Verification items for this drawing (mm, ordinates from the low corner). A direction names the side the tool comes from. Round coordinates to 2 decimals unless told otherwise and drop trailing zeros. Order: outer loops, then holes, each group sorted by start corner. A loop starts at its lowest first (then second) coordinate and runs counter-clockwise, first axis right, second up. Notation, with made-up numbers: (63, 68) -> (78, 68) arc R16 cw to (78, 73) -> close; hole circle Ø2 at (-5, 74.25). An arc over 180 degrees is marked (long way). Answer in a Markdown table with one row per item. Add a question column.
1. Material ranges on L1, parallel to X at y = 76, z = 26.5; L2, parallel to Y at x = 58, z = 7, recorded low to high. Write a range as from..to.
2. Sectioned sample at C-C, the plane z = 15. Record the boundary of the cut face in (x, y), then the cut area to 3 significant figures.
3. Depth check by flat-ended pin: P1, Ø2, axis at y = 63, z = 41, coming from the -X side; P2, Ø6.5, axis at y = 59.14, z = 20.86, coming from the +X side; P3, Ø8, axis at x = 93.5, y = 37, coming from the -Z side. Enter the tip coordinate at first touch or a pass-through.
4. Sectioned sample at D-D, the plane x = 78. Record the boundary of the cut face in (y, z).
5. Access from +Z, -Z, +X, -X, +Y, -Y to the whole of each face (thin tool, end or side, straight path). Record for the marked faces 1 and 2.
6. Sectioned sample at A-A, the plane z = 35. Record the boundary of the cut face in (x, y), then the cut area to 3 significant figures.
7. Sectioned sample at B-B, the plane y = 51.5. Record the boundary of the cut face in (x, z).
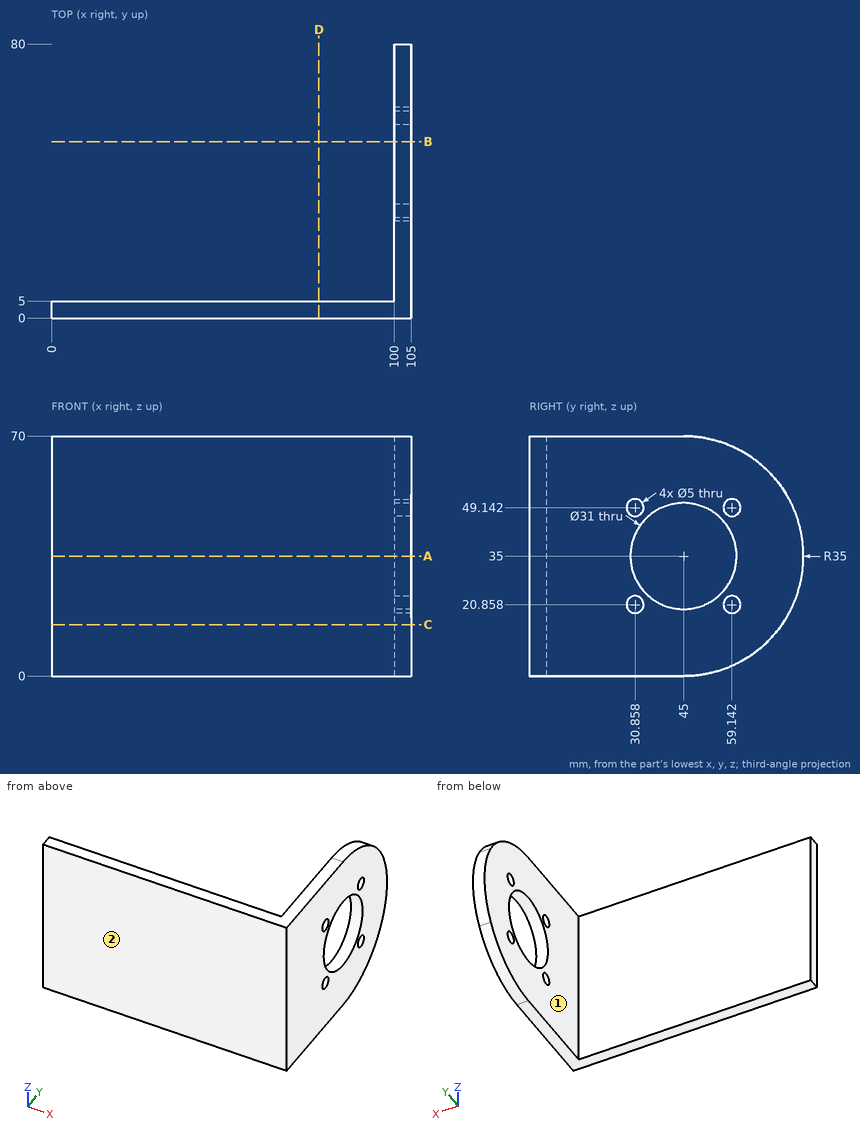
Answer key:
| question | item | result |
|---|---|---|
| 1 | L1 | x = 100..105 |
| 1 | L2 | y = 0..5 |
| 2 | outline | (0, 0) -> (105, 0) -> (105, 73.72) -> (100, 73.72) -> (100, 5) -> (0, 5) -> close |
| 2 | area | 869 mm² |
| 3 | P1 | stops at x = 100 |
| 3 | P2 | stops at x = 105 |
| 3 | P3 | passes through |
| 4 | outline | (0, 0) -> (5, 0) -> (5, 70) -> (0, 70) -> close |
| 5 | face 1 | +Z, -Z, -X, +Y |
| 5 | face 2 | +Z, -Z, +X, -X, -Y |
| 6 | outline | (0, 0) -> (105, 0) -> (105, 29.5) -> (100, 29.5) -> (100, 5) -> (0, 5) -> close; (100, 60.5) -> (105, 60.5) -> (105, 80) -> (100, 80) -> close |
| 6 | area | 745 mm² |
| 7 | outline | (100, 0.61) -> (105, 0.61) -> (105, 20.93) -> (100, 20.93) -> close; (100, 49.07) -> (105, 49.07) -> (105, 69.39) -> (100, 69.39) -> close |
